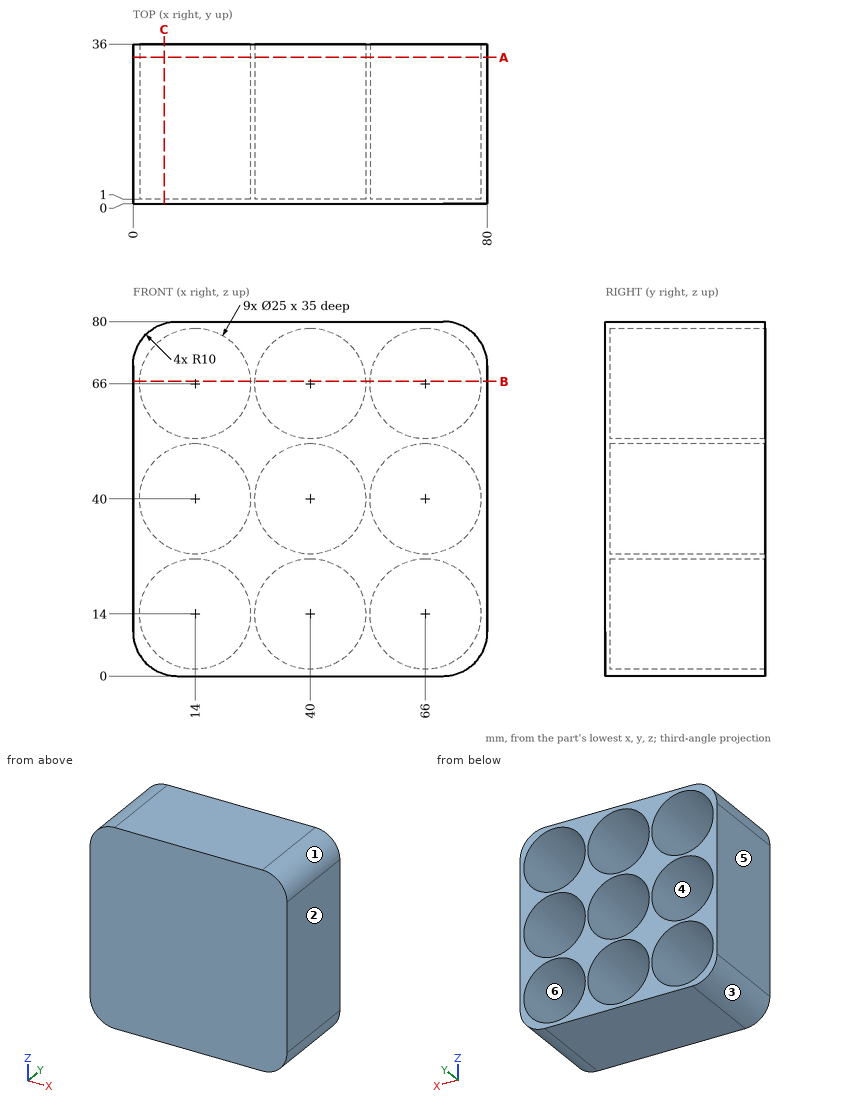
Verification items for this drawing (mm, ordinates from the low corner). A direction names the side the tool comes from. Round coordinates to 2 decimals unless told otherwise and drop trailing zeros. Loops run counter-clockwise (first coordinate to the right, second up) from the corner with the lowest first, then second, coordinate; pieces in that order, holes last. Notation, with made-up numbers: (-35.5, -35) - (-29.5, -35) arc R21 ccw to (-29.5, -19) - close; hole circle Ø3 at (69, 78). An arc over 180 degrees is marked (long way). Answer as CSV lines item,"result". Start each with the question number.
Item 1: Depth check by flat-ended pin: P1, Ø20, axis at x = 14, z = 40, coming from the +Y side. Enter the tip coordinate at first touch or a pass-through.
Item 2: Set-up check for the marked faces 5 and 6: record each of +Z, -Z, +X, -X, +Y, -Y from which the full face is reachable in a straight line by a thin tool's end or side.
Item 3: Section check A-A (y = 33). Count the separate pieces of the cut face and the enclosed holes in it, and give its area (3 significant figures).
Item 4: Scan lines: line 1 (X direction, y = 17, z = 40); line 2 (X direction, y = 35, z = 38); line 3 (Z direction, x = 76.5, y = 12.5). Record each from-to range of solid material in increasing order. Write a range as [from, to].
Item 5: Section check C-C (x = 7). Record the boundary of the cut face in (y, z), and give its area (3 significant figures).
Item 6: Section check B-B (z = 66.5). Record the boundary of the cut face in (x, y).
Item 7: Release check for a two-part mould opening along Z. For the marked faces 1, 2, 3 and 4 record: +Z half, -Z half, draft (parallel to the pull), parting line (faces both ways), or undercut.
Report:
1,P1,"stops at y = 1"
2,face 5,"+Z, -Z, -X, +Y, -Y"
2,face 6,"+Y"
3,separate pieces,"1"
3,enclosed holes,"9"
3,area,"1,900 mm2"
4,line 1,"x = [0, 1.5], [26.5, 27.5], [52.5, 53.5], [78.5, 80]"
4,line 2,"x = [0, 1.66], [26.34, 27.66], [52.34, 53.66], [78.34, 80]"
4,line 3,"z = [2.4, 7.22], [20.78, 33.22], [46.78, 59.22], [72.78, 77.6]"
5,outline,"(0, 0.46) - (36, 0.46) - (36, 3.64) - (1, 3.64) - (1, 24.36) - (36, 24.36) - (36, 29.64) - (1, 29.64) - (1, 50.36) - (36, 50.36) - (36, 55.64) - (1, 55.64) - (1, 76.36) - (36, 76.36) - (36, 79.54) - (0, 79.54) - close"
5,area,"672 mm2"
6,outline,"(0, 0) - (80, 0) - (80, 36) - (78.49, 36) - (78.49, 1) - (53.51, 1) - (53.51, 36) - (52.49, 36) - (52.49, 1) - (27.51, 1) - (27.51, 36) - (26.49, 36) - (26.49, 1) - (1.51, 1) - (1.51, 36) - (0, 36) - close"
7,face 1,"+Z half"
7,face 2,"draft"
7,face 3,"-Z half"
7,face 4,"undercut"
